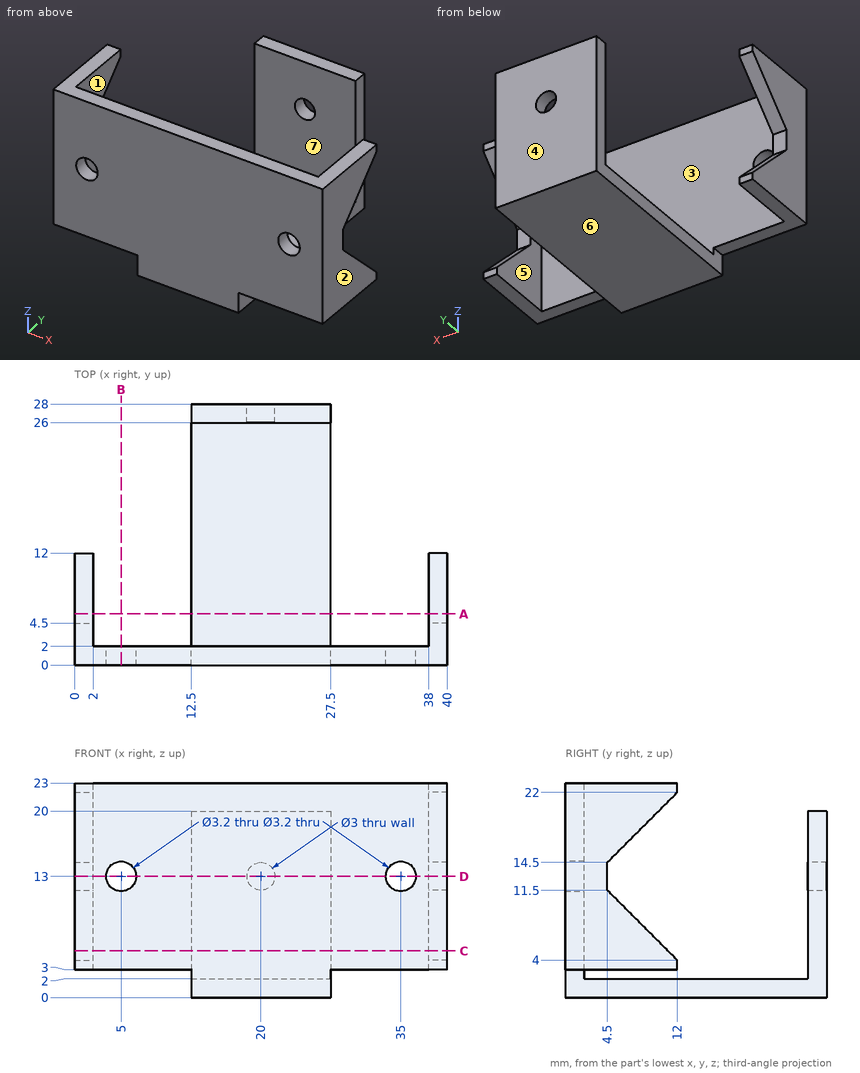
Part print with two shaded views. Sizes in mm from the minimum x, y, z corner. A direction names the side the tool comes from. Coordinates: 2 decimals unless noted, no trailing zeros. Loops run counter-clockwise (first coordinate to the right, second up) from the corner with the lowest first, then second, coordinate; pieces in that order, holes last. Notation, with made-up numbers: (10, 54.25) - (28, 54.25) arc R8 ccw to (28, 66.25) - close; hole circle Ø4 at (-5.5, 60.25). An arc over 180 degrees is marked (long way). Write each question's results on one line, items separated by ' | '. Start each with the question number.
Q1. Drop flat-ended pins along their axis: pin 1 Ø6 at (x, z) = (33, 4.5) entering from +Y; pin 2 Ø3.5 at (x, y) = (8.5, 3.5) entering from -Z; pin 3 Ø1.6 at (x, z) = (39, 13.5) entering from +Y. Give the stop position or say it passes through.
Q2. Slice it at C-C on z = 5. Give the cut face in (x, y).
Q3. Slice it at A-A on y = 5.5. Give the cut face in (x, z), and give its area (3 significant figures).
Q4. Slice it at B-B on x = 5. Give the cut face in (y, z).
Q5. Which spindle directions (+Z, -Z, +X, -X, +Y, -Y) get a long thin tool onto all of the face, cutting with end or side? Do the marked faces 5, 6 and 7. Say none if no direction does.
Q6. Slice it at D-D on z = 13. Give the cut face in (x, y), and give its area (3 significant figures).
Q7. Probe line 1 along X through (y, z) = (1.6, 13); line 2 along Y through (x, z) = (18, 2.5); line 3 along Y through (x, z) = (29, 7.5). List the from-to ranges inside material, lowest first.
Q8. Two-plate mould, pull along X, no slides. Class the marked faces 1, 2, 3 and 4: +X half, -X half, draft (parallel to the pull), parting line (faces both ways), or undercut.
Answer:
1) pin 1: stops at y = 2 | pin 2: stops at z = 3 | pin 3: stops at y = 4.5
2) outline: (0, 0) - (40, 0) - (40, 11) - (38, 11) - (38, 2) - (2, 2) - (2, 11) - (0, 11) - close; (12.5, 26) - (27.5, 26) - (27.5, 28) - (12.5, 28) - close
3) outline: (0, 3) - (2, 3) - (2, 10.5) - (0, 10.5) - close; (0, 15.5) - (2, 15.5) - (2, 23) - (0, 23) - close; (12.5, 0) - (27.5, 0) - (27.5, 2) - (12.5, 2) - close; (38, 3) - (40, 3) - (40, 10.5) - (38, 10.5) - close; (38, 15.5) - (40, 15.5) - (40, 23) - (38, 23) - close | area: 90.0 mm2
4) outline: (0, 3) - (2, 3) - (2, 11.4) - (0, 11.4) - close; (0, 14.6) - (2, 14.6) - (2, 23) - (0, 23) - close
5) face 5: +Z, -Z, +Y | face 6: -Z, +X, -X, +Y, -Y | face 7: +Z, +X, -X
6) outline: (0, 0) - (3.4, 0) - (3.4, 2) - (2, 2) - (2, 4.5) - (0, 4.5) - close; (6.6, 0) - (33.4, 0) - (33.4, 2) - (6.6, 2) - close; (12.5, 26) - (18.5, 26) - (18.5, 28) - (12.5, 28) - close; (21.5, 26) - (27.5, 26) - (27.5, 28) - (21.5, 28) - close; (36.6, 0) - (40, 0) - (40, 4.5) - (38, 4.5) - (38, 2) - (36.6, 2) - close | area: 101 mm2
7) line 1: x = 0 to 3.4, 6.6 to 33.4, 36.6 to 40 | line 2: y = 0 to 2, 26 to 28 | line 3: y = 0 to 2
8) face 1: undercut | face 2: +X half | face 3: undercut | face 4: draft
